Build history of the part. All positions in model axes, mm. Face numbers are marked on the shaded views. Give positions to 0.01 mm unless a question says otherwise; leave off trailing zeros. Write each loop counter-clockwise with the first axis right and the second up, starting at its lowest first coordinate (ties: lowest second). Pieces come first, ordered by that corner, then holes. Notation, with made-up numbers: M -5.5,-28 L 29.5,-28 A11 cw 29.5,-9 Z; hole C -28.5,88 d10. An arc over 180 degrees is marked long. Return JSON: item names as keys, results as strings. Group by question number.
Q1. Band-saw the part on B-B, the plane y = -9. Give the cut face in (x, z).
Q2. Pull direction Z, two halves, no side cores. Call the marked faces 1 and 2: +Z half, -Z half, draft (parallel to the pull), parting line (faces both ways), or undercut.
Q3. Band-saw the part on C-C, the plane x = -311.5. Give the cut face in (y, z).
Q4. Band-saw the part on A-A, the plane z = 0. Give the cut face in (x, y), then the cut area to 3 significant figures.
Q5. Flat gauge pins, fed straight in: pin 1 Ø8 at (x, y) = (-637.5, -33) entering from +Z; pin 2 Ø12 at (x, y) = (-249.5, -9) entering from -Z; pin 3 Ø12 at (x, y) = (-736, -35) entering from +Z. Where does each tip first touch, or does it go through?
Q6. Wall check: probe 1 along Z at (x, y) = (-536, -25); probe 2 along Z at (x, y) = (-178, -2.5); probe 3 along X at (y, z) = (-21, -10.5). Give the ranges that are in metal, low to high.
from build123d import *

# Parameters (mm, degrees)
F1_DEPTH = 60


with BuildPart() as f1:
    # F0 (on Front) → F1 (new body)
    with BuildSketch(Plane.XZ):
        with BuildLine():
            Line((0, -150), (0, 0))
            Line((0, 0), (0, 150))
            Line((0, 150), (-729.295073, 124.926188))
            ThreePointArc((-729.295073, 124.926188), (-850, 0), (-729.295073, -124.926188))
            Line((-729.295073, -124.926188), (0, -150))
        make_face()
        with BuildLine():
            Line((-1.5, 148.447542), (-1.5, 0))
            Line((-1.5, 0), (-1.5, -148.447542))
            Line((-1.5, -148.447542), (-729.243532, -123.427073))
            ThreePointArc((-729.243532, -123.427073), (-848.5, 0), (-729.243532, 123.427073))
            Line((-729.243532, 123.427073), (-1.5, 148.447542))
        make_face(mode=Mode.SUBTRACT)
    extrude(amount=F1_DEPTH)


solid = f1.part
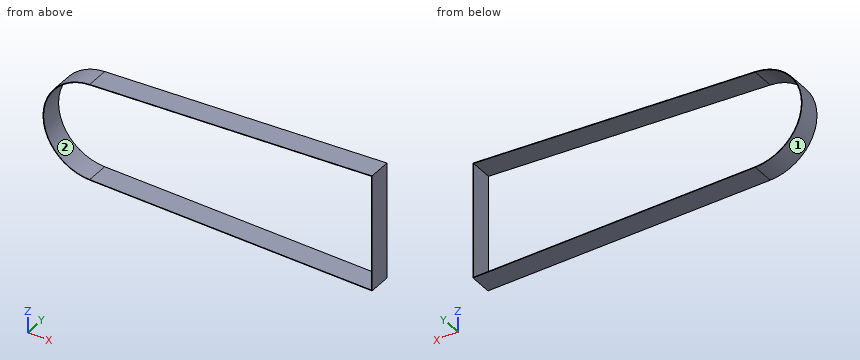
From the geometry:
{
 "1": {"outline": "M -729.3,-124.93 L 0,-150 L 0,150 L -729.3,124.93 A125 ccw Z; hole M -729.24,-123.43 L -1.5,-148.45 L -1.5,148.45 L -729.24,123.43 A123.5 ccw Z"},
 "2": {"face 1": "parting line", "face 2": "undercut"},
 "3": {"outline": "M -60,-139.29 L 0,-139.29 L 0,-137.79 L -60,-137.79 Z; M -60,137.79 L 0,137.79 L 0,139.29 L -60,139.29 Z"},
 "4": {"outline": "M -850,-60 L -848.5,-60 L -848.5,0 L -850,0 Z; M -1.5,-60 L 0,-60 L 0,0 L -1.5,0 Z", "area": "180 mm^2"},
 "5": {"pin 1": "stops at z = 128.22", "pin 2": "stops at z = -141.63", "pin 3": "stops at z = 124.9"},
 "6": {"probe 1": "z = -131.57 to -130.07, 130.07 to 131.57", "probe 2": "z = -143.88 to -142.38, 142.38 to 143.88", "probe 3": "x = -849.56 to -848.05, -1.5 to 0"}
}
